Geometry: final body of the model. Coordinates: model frame, mm. Give positions to 0.01 mm unless a question says otherwise; leave off trailing zeros. Write each loop counter-clockwise with the first axis right and the second up, starting at its lowest first coordinate (ties: lowest second). Pieces come first, ordered by that corner, then holes. Notation, with made-up numbers: (64, -10) - (72, -10) arc R27 cw to (72, 26) - close; hole circle Ø7 at (53.5, 38). An arc over 180 degrees is marked (long way). Use CSV: the item, a comma, the result in double quotes. Start each with the question number.
(1) First-contact query: pin 1 Ø1.5 at (x, z) = (36.5, 2) entering from -Y; pin 2 Ø2.5 at (x, z) = (35, 3.5) entering from +Y. Flat tips, straight axial feed; report the tip coordinate or a pass-through.
(2) Line query: probe 1 along Y at (x, z) = (48, 2.2); probe 2 along Y at (x, z) = (40.5, 4.4); probe 3 along X at (y, z) = (212, 2). Output: solid intervals per line, ascending. Write a range as [from, to].
(3) Section C-C on z = 1.8. Count the separate pieces of the cut face and the enclosed holes in it, and give its area (3 significant figures).
(4) Section B-B on y = 150. Output: boundary loops of the cut face in (x, z), and give its area (3 significant figures).
(5) Section D-D on y = 214. Output: boundary loops of the cut face in (x, z), and give its area (3 significant figures).
(6) Section A-A on x = 56. Output: boundary loops of the cut face in (y, z), and give its area (3 significant figures).
from build123d import *

# Parameters (mm, degrees)
SKETCH_1_W          = 25
SKETCH_1_H          = 5
SKETCH_1_W_2        = 70
SKETCH_1_H_2        = 190
EXTRUDE_1_DEPTH     = 5
SKETCH_2_R          = 1.55
CUT_EXTRUDE_1_DEPTH = 5
SKETCH_3_W          = 25
SKETCH_3_H          = 70
EXTRUDE_2_DEPTH     = 5
SKETCH_4_W          = 50
SKETCH_4_H          = 72.5
CUT_EXTRUDE_2_DEPTH = 5
FILLET_1_R          = 10
FILLET_2_R          = 1


with BuildPart() as part:
    # 草图1 → 凸台-拉伸1 (new body)
    with BuildSketch(Plane.XY):
        with Locations((57.5, 192.5)):
            Rectangle(SKETCH_1_W, SKETCH_1_H)
        with Locations((35, 95)):
            Rectangle(SKETCH_1_W_2, SKETCH_1_H_2)
        with Locations((12.5, 192.5)):
            Rectangle(SKETCH_1_W, SKETCH_1_H)
        with Locations((57.5, -2.5)):
            Rectangle(SKETCH_1_W, SKETCH_1_H)
        with Locations((12.5, -2.5)):
            Rectangle(SKETCH_1_W, SKETCH_1_H)
    extrude(amount=EXTRUDE_1_DEPTH)

    # 草图2 → 切除-拉伸1 (cut)
    with BuildSketch(Plane.XY.offset(5)):
        with Locations((43.45, 0)):
            Circle(SKETCH_2_R)
        with Locations((26.55, 0)):
            Circle(SKETCH_2_R)
        with Locations((43.45, 190)):
            Circle(SKETCH_2_R)
        with Locations((26.55, 190)):
            Circle(SKETCH_2_R)
    extrude(amount=-CUT_EXTRUDE_1_DEPTH, mode=Mode.SUBTRACT)

    # 草图3 → 凸台-拉伸2 (add)
    with BuildSketch(Plane.XY.offset(5)):
        with Locations((12.5, 230)):
            Rectangle(SKETCH_3_W, SKETCH_3_H)
        with Locations((57.5, 230)):
            Rectangle(SKETCH_3_W, SKETCH_3_H)
    extrude(amount=-EXTRUDE_2_DEPTH)

    # 草图4 → 切除-拉伸2 (cut)
    with BuildSketch(Plane.XY.offset(5)):
        with Locations((35, 138.75)):
            Rectangle(SKETCH_4_W, SKETCH_4_H)
        with Locations((35, 51.25)):
            Rectangle(SKETCH_4_W, SKETCH_4_H)
    extrude(amount=-CUT_EXTRUDE_2_DEPTH, mode=Mode.SUBTRACT)

    # 圆角1
    fillet_1_edges = [part.edges().sort_by_distance(p)[0] for p in [
        (10, 15, 2.5),
        (10, 87.5, 2.5),
        (60, 87.5, 2.5),
        (60, 15, 2.5),
        (60, 102.5, 2.5),
        (10, 102.5, 2.5),
        (10, 175, 2.5),
        (60, 175, 2.5),
    ]]
    fillet(fillet_1_edges, radius=FILLET_1_R)

    # 圆角2
    fillet_2_edges = [part.edges().sort_by_distance(p)[0] for p in [
        (70, -5, 2.5),
        (45, -5, 2.5),
        (25, -5, 2.5),
        (0, -5, 2.5),
        (25, 265, 2.5),
        (0, 265, 2.5),
        (70, 265, 2.5),
        (45, 265, 2.5),
    ]]
    fillet(fillet_2_edges, radius=FILLET_2_R)


solid = part.part
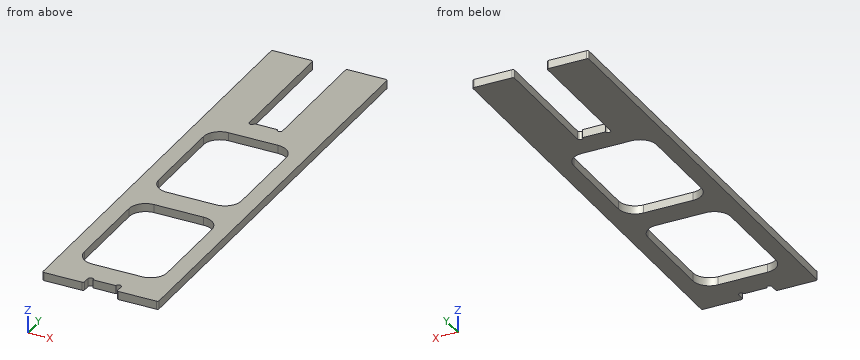
Check values:
1,pin 1,"stops at y = 0"
1,pin 2,"stops at y = 190"
2,probe 1,"y = [-5, 15], [87.5, 102.5], [175, 265]"
2,probe 2,"y = [0, 15], [87.5, 102.5], [175, 190]"
2,probe 3,"x = [0, 25], [45, 70]"
3,separate pieces,"1"
3,enclosed holes,"2"
3,area,"10,200 mm²"
4,outline,"(0, 0) - (10, 0) - (10, 5) - (0, 5) - close; (60, 0) - (70, 0) - (70, 5) - (60, 5) - close"
4,area,"100 mm²"
5,outline,"(0, 0) - (25, 0) - (25, 5) - (0, 5) - close; (45, 0) - (70, 0) - (70, 5) - (45, 5) - close"
5,area,"250 mm²"
6,outline,"(-5, 0) - (17, 0) - (17, 5) - (-5, 5) - close; (85.5, 0) - (104.5, 0) - (104.5, 5) - (85.5, 5) - close; (173, 0) - (265, 0) - (265, 5) - (173, 5) - close"
6,area,"665 mm²"
